from build123d import *

# Parameters (mm, degrees)
SKETCH2_R           = 60
SKETCH2_R_2         = 47.5
BOSS_EXTRUDE2_DEPTH = 10


with BuildPart() as part:
    # Sketch2 → Boss-Extrude2 (new body)
    with BuildSketch(Plane.XY):
        Polygon((10.635083269, 120), (10.635083269, 135), (-444.364916731, 135), (-444.364916731, 120), (-449.364916731, 120), (-449.364916731, 35), (-430, 0), (0, 0), (15.635083269, 35), (15.635083269, 120), align=None)
        with Locations((-160, 70)):
            Circle(SKETCH2_R, mode=Mode.SUBTRACT)
        with Locations((-305, 70)):
            Circle(SKETCH2_R, mode=Mode.SUBTRACT)
        with Locations((-160, 70)):
            Circle(SKETCH2_R)
        with Locations((-160, 70)):
            Circle(SKETCH2_R_2, mode=Mode.SUBTRACT)
        with Locations((-305, 70)):
            Circle(SKETCH2_R)
        with Locations((-305, 70)):
            Circle(SKETCH2_R_2, mode=Mode.SUBTRACT)
    extrude(amount=BOSS_EXTRUDE2_DEPTH)


solid = part.part
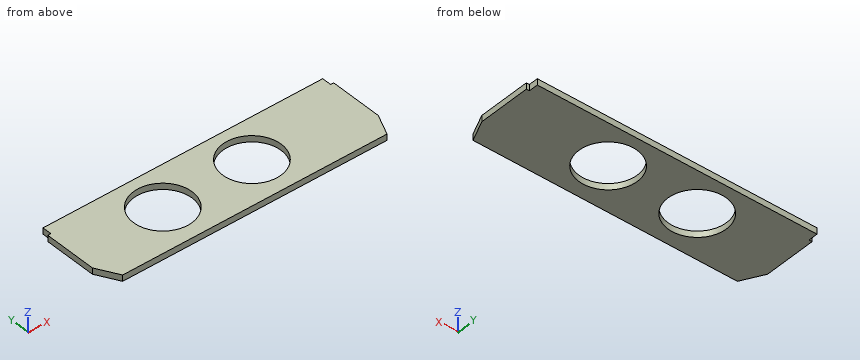
Geometry: final body of the model. Coordinates: model frame, mm. Coordinates: 2 decimals unless noted, no trailing zeros. Order: outer loops, then holes, each group sorted by start corner. A loop starts at its lowest first (then second) coordinate and runs counter-clockwise, first axis right, second up. Notation, with made-up numbers: M 84,51 L 142,51 A23 cw 142,75 Z; hole C 29.5,-7 d6. An arc over 180 degrees is marked long. One line per question, with ' | ' between items. Start each with the question number.
Item 1: Pin query (flat end, axial travel): pin 1 Ø5 at (y, z) = (124.5, 4) entering from -X; pin 2 Ø2 at (y, z) = (21.5, 6) entering from -X; pin 3 Ø2.5 at (x, z) = (-446.5, 4) entering from +Y. Return the tip coordinate at first contact, or that it passes through.
Item 2: Cut plane C-C, the plane z = 3.5. Return the cut outline in (x, y).
Item 3: Cut plane B-B, the plane y = 70. Return the cut outline in (x, z), then the cut area to 3 significant figures.
Item 4: Cut plane D-D, the plane y = 39. Return the cut outline in (x, z).
Item 5: Cut plane A-A, the plane x = -160. Return the cut outline in (y, z), then the cut area to 3 significant figures.
Item 6: Ray query, probe 1 along Y at (x, z) = (-160, 6.75); probe 2 along X at (y, z) = (28, 2.25); probe 3 along X at (y, z) = (99, 1.5). Return the intervals inside material, ascending. Write a range as [from, to].
A:
1) pin 1: stops at x = -444.36 | pin 2: stops at x = -442.45 | pin 3: stops at y = 120
2) outline: M -449.36,35 L -430,0 L 0,0 L 15.64,35 L 15.64,120 L 10.64,120 L 10.64,135 L -444.36,135 L -444.36,120 L -449.36,120 Z; hole C -305,70 d95; hole C -160,70 d95
3) outline: M -449.36,0 L -352.5,0 L -352.5,10 L -449.36,10 Z; M -257.5,0 L -207.5,0 L -207.5,10 L -257.5,10 Z; M -112.5,0 L 15.64,0 L 15.64,10 L -112.5,10 Z | area: 2,750 mm2
4) outline: M -449.36,0 L -340.99,0 L -340.99,10 L -449.36,10 Z; M -269.01,0 L -195.99,0 L -195.99,10 L -269.01,10 Z; M -124.01,0 L 15.64,0 L 15.64,10 L -124.01,10 Z
5) outline: M 0,0 L 22.5,0 L 22.5,10 L 0,10 Z; M 117.5,0 L 135,0 L 135,10 L 117.5,10 Z | area: 400 mm2
6) probe 1: y = [0, 22.5], [117.5, 135] | probe 2: x = [-445.49, -327.19], [-282.81, -182.19], [-137.81, 12.51] | probe 3: x = [-449.36, -342.62], [-267.38, -197.62], [-122.38, 15.64]
